```python
from build123d import *

# Parameters (mm, degrees)
BOSS_EXTRUDE1_DEPTH = 1.524


with BuildPart() as part:
    # Sketch1 → Boss-Extrude1 (new body)
    with BuildSketch(Plane.XY):
        with BuildLine():
            Line((243.009394749, 226.483628693), (252.19647472, 225.051376489))
            ThreePointArc((252.19647472, 225.051376489), (252.501172451, 224.932897548), (252.728179767, 224.697640997))
            ThreePointArc((252.728179767, 224.697640997), (253.158948075, 219.940008266), (255.562248507, 215.811476133))
            ThreePointArc((255.562248507, 215.811476133), (251.141222731, 217.242232573), (246.682055702, 218.549275922))
            Line((246.682055702, 218.549275922), (232.141476548, 226.101345829))
            Line((232.141476548, 226.101345829), (212.521244057, 231.994935761))
            Line((212.521244057, 231.994935761), (233.004487141, 231.64183795))
            Line((233.004487141, 231.64183795), (249.153153432, 234.413620597))
            ThreePointArc((249.153153432, 234.413620597), (253.798600989, 234.302490495), (258.445341479, 234.320813134))
            ThreePointArc((258.445341479, 234.320813134), (254.900209484, 231.11883411), (253.042819444, 226.717614645))
            ThreePointArc((253.042819444, 226.717614645), (252.755013662, 226.562547569), (252.428715894, 226.542355168))
            Line((252.428715894, 226.542355168), (243.241260726, 227.972198625))
            Line((243.241260726, 227.972198625), (243.009394749, 226.483628693))
        make_face()
    extrude(amount=BOSS_EXTRUDE1_DEPTH)


solid = part.part
```
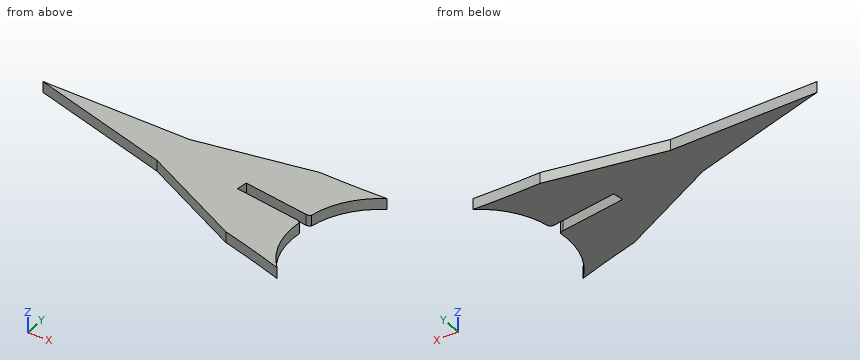
Read the model definition and answer for the solid it produces. Units are mm, in the model's axes. Coordinates: 2 decimals unless noted, no trailing zeros. Order: outer loops, then holes, each group sorted by start corner. A loop starts at its lowest first (then second) coordinate and runs counter-clockwise, first axis right, second up. Notation, with made-up numbers: (48, 25) - (75, 25) arc R23 ccw to (75, 54) - close; hole circle Ø1 at (-40, -11). An arc over 180 degrees is marked (long way). Answer as a JSON object with one key per item and string values. Group by question number.
Item 1: A flat-ended cylindrical pin translates along its axis: P1, Ø1, axis at x = 243.5, y = 222.5, coming from the -Z side. Find the tip coordinate at first contact, or state that the pin passes through.
Item 2: Section C-C (y = 217.5) is taken. Give the vertices of the cut face in (x, z), plus the area to 3 significant figures.
Item 3: Section D-D (x = 242) is taken. Give the vertices of the cut face in (y, z).
Item 4: Consider probe 1 along Y at (x, z) = (244, 0.75); probe 2 along Y at (x, z) = (248, 1); probe 3 along X at (y, z) = (224, 1.1). Determine where each line is inside the solid, lowest interval first. Write a range as from..to.
Item 5: Section B-B (z = 1.1) is taken. Give the vertices of the cut face in (x, y), plus the area to 3 significant figures.
Item 6: Section A-A (x = 250) is taken. Give the vertices of the cut face in (y, z).
Results are:
{
 "1": {"P1": "stops at z = 0"},
 "2": {"outline": "(250.3, 0) - (254.28, 0) - (254.28, 1.52) - (250.3, 1.52) - close", "area": "6.07 mm^2"},
 "3": {"outline": "(220.98, 0) - (233.19, 0) - (233.19, 1.52) - (220.98, 1.52) - close"},
 "4": {"probe 1": "y = 219.94..226.33, 227.85..233.53", "probe 2": "y = 218.18..225.71, 227.23..234.22", "probe 3": "x = 236.19..252.66"},
 "5": {"outline": "(212.52, 231.99) - (232.14, 226.1) - (246.68, 218.55) arc R166.79 cw to (255.56, 215.81) arc R11.02 cw to (252.73, 224.7) arc R0.76 ccw to (252.2, 225.05) - (243.01, 226.48) - (243.24, 227.97) - (252.43, 226.54) arc R0.76 ccw to (253.04, 226.72) arc R11.02 cw to (258.45, 234.32) arc R166.79 cw to (249.15, 234.41) - (233, 231.64) - close", "area": "313 mm^2"},
 "6": {"outline": "(217.59, 0) - (225.39, 0) - (225.39, 1.52) - (217.59, 1.52) - close; (226.92, 0) - (234.38, 0) - (234.38, 1.52) - (226.92, 1.52) - close"}
}
